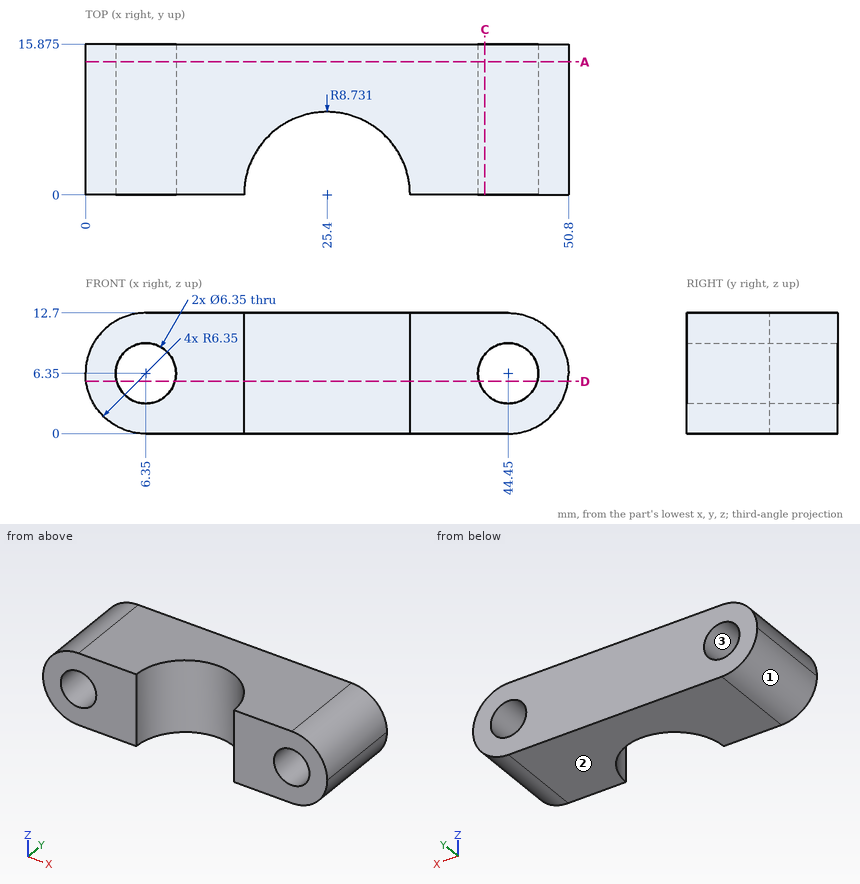
Answer from the drawing. Dimensions are ordinates in mm from the lowest x, y and z of the part. Round coordinates to 2 decimals unless told otherwise and drop trailing zeros. Loops run counter-clockwise (first coordinate to the right, second up) from the corner with the lowest first, then second, coordinate; pieces in that order, holes last. Notation, with made-up numbers: (-12.5, 23.5) - (13.5, 23.5) arc R22 ccw to (13.5, 40.5) - close; hole circle Ø11 at (80.25, 26.25). An arc over 180 degrees is marked (long way). One line per item, written item: value.
Q1. Each of these flat-tipped pins is pushed along its axis until it touches: pin 1 Ø1 at (x, z) = (33, 9.5) entering from -Y; pin 2 Ø4 at (y, z) = (13.5, 2) entering from +X. Where does it stop, or does it pass through?
Check values:
pin 1: y = 3.26
pin 2: x = 50.35
Q2. Straight lines are drawn through the part: probe 1 along X at (y, z) = (9.5, 6.35) (1 decimal); probe 2 along Z at (x, y) = (6.35, 6.5) (1 decimal); probe 3 along X at (y, z) = (2.25, 3.75) (1 decimal). For each, find the intervals that lie inside material, in ascending order.
Check values:
probe 1: 0 to 3.2, 9.5 to 41.3, 47.6 to 50.8
probe 2: 0 to 3.2, 9.5 to 12.7
probe 3: 0.6 to 4.5, 8.2 to 17, 33.8 to 42.6, 46.3 to 50.2
Q3. Find section D-D on z = 5.5. Give the vertices of the cut face in (x, y) (1 decimal), and give its area (3 significant figures).
Check values:
outline: (0.1, 0) - (3.3, 0) - (3.3, 15.9) - (0.1, 15.9) - close; (9.4, 0) - (16.7, 0) arc R8.7 cw to (34.1, 0) - (41.4, 0) - (41.4, 15.9) - (9.4, 15.9) - close; (47.5, 0) - (50.7, 0) - (50.7, 15.9) - (47.5, 15.9) - close
area: 491 mm2
Q4. Find section A-A on y = 14. State how many separate pieces and enclosed holes the cut face has, and give its area (3 significant figures).
Check values:
separate pieces: 1
enclosed holes: 2
area: 547 mm2
Q5. The mould has two halves that part along X. Classify the marked faces 1, 2 and 3: +X half, -X half, draft (parallel to the pull), parting line (faces both ways), or undercut.
Check values:
face 1: -X half
face 2: draft
face 3: undercut
Q6. Find section C-C on x = 42. Give the vertices of the cut face in (y, z) (1 decimal), and give its area (4 significant figures).
Check values:
outline: (0, 0) - (15.9, 0) - (15.9, 4.3) - (0, 4.3) - close; (0, 8.4) - (15.9, 8.4) - (15.9, 12.7) - (0, 12.7) - close
area: 137.5 mm2
